from build123d import *

# Parameters (mm, degrees)
BOSS_EXTRUDE5_DEPTH = 1.5875


with BuildPart() as part:
    # carrier → Boss-Extrude5 (new body)
    with BuildSketch(Plane(origin=(-89.612357323, 67.458483608, 0), x_dir=(1, 0, 0), z_dir=(0, 0, 1))):
        with BuildLine():
            Line((118.819010038, 161.989326691), (118.810191038, 161.980520691))
            Line((118.810191038, 161.980520691), (125.512969038, 150.382951691))
            Line((125.512969038, 150.382951691), (118.819010038, 138.794201691))
            Line((118.819010038, 138.794201691), (118.810191038, 138.776562691))
            add(Edge.make_bspline(
                [(118.810191038, 138.776562691), (118.138894038, 137.665721691), (117.760677038, 136.367990691), (117.760677038, 134.975382691)],
                knots=[0, 0, 0, 0, 1, 1, 1, 1], degree=3))
            add(Edge.make_bspline(
                [(117.760677038, 134.975382691), (117.760675038, 130.905661691), (121.064010038, 127.602323691), (125.133733038, 127.602326691)],
                knots=[0, 0, 0, 0, 1, 1, 1, 1], degree=3))
            add(Edge.make_bspline(
                [(125.133733038, 127.602326691), (127.909953038, 127.602326691), (130.315556038, 129.144498691), (131.571927038, 131.412326691)],
                knots=[0, 0, 0, 0, 1, 1, 1, 1], degree=3))
            Line((131.571927038, 131.412326691), (131.580732038, 131.403521691))
            Line((131.580732038, 131.403521691), (138.283510038, 143.009910691))
            Line((138.283510038, 143.009910691), (151.653788038, 143.009910691))
            Line((151.653788038, 143.009910691), (151.671427038, 143.009910691))
            add(Edge.make_bspline(
                [(151.671427038, 143.009910691), (152.969090038, 142.983973691), (154.284212038, 143.301383691), (155.490246038, 143.997687691)],
                knots=[0, 0, 0, 0, 1, 1, 1, 1], degree=3))
            add(Edge.make_bspline(
                [(155.490246038, 143.997687691), (159.014728038, 146.032549691), (160.223858038, 150.545012691), (158.188996038, 154.069493691)],
                knots=[0, 0, 0, 0, 1, 1, 1, 1], degree=3))
            add(Edge.make_bspline(
                [(158.188996038, 154.069493691), (156.800886038, 156.473769691), (154.263610038, 157.793065691), (151.671427038, 157.747201691)],
                knots=[0, 0, 0, 0, 1, 1, 1, 1], degree=3))
            Line((151.671427038, 157.747201691), (151.671427038, 157.754849091))
            Line((151.671427038, 157.754849091), (138.224971754, 157.754849091))
            Line((138.224971754, 157.754849091), (131.539832754, 169.334779091))
            Line((131.539832754, 169.334779091), (131.531027754, 169.352418091))
            add(Edge.make_bspline(
                [(131.531027754, 169.352418091), (130.904660754, 170.489198091), (129.976575754, 171.469517091), (128.770540754, 172.165821091)],
                knots=[0, 0, 0, 0, 1, 1, 1, 1], degree=3))
            add(Edge.make_bspline(
                [(128.770540754, 172.165821091), (127.565708199, 172.861433534), (126.244241887, 173.179504317), (124.946928377, 173.154056045)],
                knots=[0, 0, 0, 0, 0.994463703, 0.994463703, 0.994463703, 0.994463703], degree=3))
            add(Edge.make_bspline(
                [(124.946928377, 173.154056045), (122.467005204, 173.088633853), (120.078815068, 171.772470761), (118.748455038, 169.468215691)],
                knots=[0.003756223, 0.003756223, 0.003756223, 0.003756223, 1, 1, 1, 1], degree=3))
            add(Edge.make_bspline(
                [(118.748455038, 169.468215691), (117.360345038, 167.063938691), (117.483199038, 164.211290691), (118.819010038, 161.989326691)],
                knots=[0, 0, 0, 0, 1, 1, 1, 1], degree=3))
        make_face()
        with BuildLine():
            Line((131.348201, 148.224924), (136.683962, 148.224924))
            add(Edge.make_bspline(
                [(136.683962, 148.224924), (137.161645, 148.814777), (137.451253, 149.56754), (137.451253, 150.385688)],
                knots=[0, 0, 0, 0, 1, 1, 1, 1], degree=3))
            add(Edge.make_bspline(
                [(137.451253, 150.385688), (137.451253, 151.203836), (137.161645, 151.94778), (136.683962, 152.537633)],
                knots=[0, 0, 0, 0, 1, 1, 1, 1], degree=3))
            Line((136.683962, 152.537633), (131.348201, 152.537633))
            add(Edge.make_bspline(
                [(131.348201, 152.537633), (130.870517, 151.94778), (130.580909, 151.203836), (130.580909, 150.385688)],
                knots=[0, 0, 0, 0, 1, 1, 1, 1], degree=3))
            add(Edge.make_bspline(
                [(130.580909, 150.385688), (130.580909, 149.56754), (130.870517, 148.814777), (131.348201, 148.224924)],
                knots=[0, 0, 0, 0, 1, 1, 1, 1], degree=3))
        make_face(mode=Mode.SUBTRACT)
        with BuildLine():
            add(Edge.make_bspline(
                [(154.547076, 150.381274), (154.547076, 148.865969), (153.318678, 147.637574), (151.803377, 147.637574)],
                knots=[0, 0, 0, 0, 1, 1, 1, 1], degree=3))
            add(Edge.make_bspline(
                [(151.803377, 147.637574), (150.288072, 147.637574), (149.059677, 148.865969), (149.059677, 150.381274)],
                knots=[0, 0, 0, 0, 1, 1, 1, 1], degree=3))
            add(Edge.make_bspline(
                [(149.059677, 150.381274), (149.059677, 151.896576), (150.288072, 153.124973), (151.803377, 153.124973)],
                knots=[0, 0, 0, 0, 1, 1, 1, 1], degree=3))
            add(Edge.make_bspline(
                [(151.803377, 153.124973), (153.318678, 153.124973), (154.547076, 151.896576), (154.547076, 150.381274)],
                knots=[0, 0, 0, 0, 1, 1, 1, 1], degree=3))
        make_face(mode=Mode.SUBTRACT)
        with BuildLine():
            add(Edge.make_bspline(
                [(123.750123, 168.162095), (125.062416, 168.919747), (126.740436, 168.470121), (127.498087, 167.157831)],
                knots=[0, 0, 0, 0, 1, 1, 1, 1], degree=3))
            add(Edge.make_bspline(
                [(127.498087, 167.157831), (128.255739, 165.845539), (127.806115, 164.16752), (126.493823, 163.409868)],
                knots=[0, 0, 0, 0, 1, 1, 1, 1], degree=3))
            add(Edge.make_bspline(
                [(126.493823, 163.409868), (125.181533, 162.652217), (123.503512, 163.101839), (122.74586, 164.414132)],
                knots=[0, 0, 0, 0, 1, 1, 1, 1], degree=3))
            add(Edge.make_bspline(
                [(122.74586, 164.414132), (121.988209, 165.726422), (122.437834, 167.404444), (123.750123, 168.162095)],
                knots=[0, 0, 0, 0, 1, 1, 1, 1], degree=3))
        make_face(mode=Mode.SUBTRACT)
        with BuildLine():
            add(Edge.make_bspline(
                [(123.750127, 132.600451), (122.437834, 133.358103), (121.988212, 135.036124), (122.745863, 136.348414)],
                knots=[0, 0, 0, 0, 1, 1, 1, 1], degree=3))
            add(Edge.make_bspline(
                [(122.745863, 136.348414), (123.503515, 137.660706), (125.181534, 138.11033), (126.493826, 137.352678)],
                knots=[0, 0, 0, 0, 1, 1, 1, 1], degree=3))
            add(Edge.make_bspline(
                [(126.493826, 137.352678), (127.806116, 136.595027), (128.255742, 134.917007), (127.49809, 133.604715)],
                knots=[0, 0, 0, 0, 1, 1, 1, 1], degree=3))
            add(Edge.make_bspline(
                [(127.49809, 133.604715), (126.740439, 132.292425), (125.062417, 131.8428), (123.750127, 132.600451)],
                knots=[0, 0, 0, 0, 1, 1, 1, 1], degree=3))
        make_face(mode=Mode.SUBTRACT)
    extrude(amount=BOSS_EXTRUDE5_DEPTH)


solid = part.part
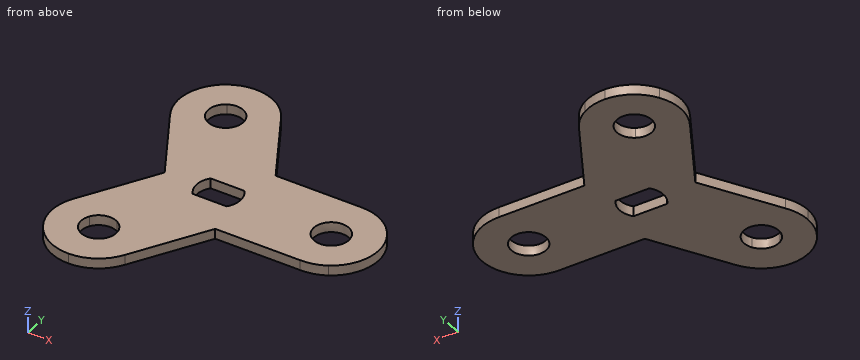
Build history of the part. All positions in model axes, mm. Coordinates: 2 decimals unless noted, no trailing zeros. Write each loop counter-clockwise with the first axis right and the second up, starting at its lowest first coordinate (ties: lowest second). Pieces come first, ordered by that corner, then holes.
(1) Drill centre lines: line 1 (Y direction, x = 61, z = 0.95); line 2 (Y direction, x = 56, z = 0.8); line 3 (Y direction, x = 43, z = 0.1). Where is each one in solid material? Low to high.
(2) Cut at A-A on x = 42.5. List the corners of the cut face in (y, z), and give its area (3 significant figures).
(3) Cut at D-D on y = 208. List the corners of the cut face in (x, z).
(4) Pin check, flat tips, straight feed: pin 1 Ø2 at (x, y) = (32.5, 218.5) entering from +Z; pin 2 Ø0.8 at (x, z) = (45, 0.5) entering from -Y. Stop position of each tip, or through.
(5) Cut at C-C on z = 0.3. State how many separate pieces and enclosed holes the cut face has, and give its area (3 significant figures).
(6) Cut at B-B on x = 58. List the corners of the cut face in (y, z), and give its area (3 significant figures).
Working result:
1. line 1: y = 210.47 to 215.37, 220.31 to 225.21
1. line 2: y = 210.47 to 225.21
1. line 3: y = 200.65 to 215.68, 220 to 234.94
2. outline: (199.78, 0) - (215.68, 0) - (215.68, 1.59) - (199.78, 1.59) - close; (220, 0) - (235.8, 0) - (235.8, 1.59) - (220, 1.59) - close
2. area: 50.3 mm2
3. outline: (30.22, 0) - (47.25, 0) - (47.25, 1.59) - (30.22, 1.59) - close
4. pin 1: passes through
4. pin 2: stops at y = 203.42
5. separate pieces: 1
5. enclosed holes: 4
5. area: 849 mm2
6. outline: (210.47, 0) - (225.21, 0) - (225.21, 1.59) - (210.47, 1.59) - close
6. area: 23.4 mm2
